from build123d import *

# Parameters (mm, degrees)
F0_R     = 26.4876043929
F1_DEPTH = 14.732
F2_SIZE  = 2.54
F3_R     = 21.3384472315
F4_DEPTH = 3.048
F4_TAPER = 30
F5_R     = 5.08


with BuildPart() as f1:
    # F0 (on Top) → F1 (new body)
    with BuildSketch(Plane.XY):
        Circle(F0_R)
    extrude(amount=F1_DEPTH)

    # F2
    f2_edges = [f1.edges().sort_by_distance(p)[0] for p in [
        (-26.487604, 0, 14.732),
    ]]
    chamfer(f2_edges, length=F2_SIZE)

    # F3 (on face) → F4 (join)
    with BuildSketch(Plane.XY.offset(14.732)):
        Circle(F3_R)
    extrude(amount=F4_DEPTH, taper=F4_TAPER)

    # F5
    f5_edges = [f1.edges().sort_by_distance(p)[0] for p in [
        (-19.578684, 0, 17.78),
    ]]
    fillet(f5_edges, radius=F5_R)


solid = f1.part
Design review of the part built by this model. Coordinates are the model's own, in mm. A direction names the side the tool comes from. Give positions to 0.01 mm unless a question says otherwise; leave off trailing zeros. Loops run counter-clockwise (first coordinate to the right, second up) from the corner with the lowest first, then second, coordinate; pieces in that order, holes last. Notation, with made-up numbers: M -3,-27.5 L 31,-27.5 A20 ccw 31,-18.5 Z; hole C 49.5,-9 d4. An arc over 180 degrees is marked long. One line per question, with ' | ' between items. Start each with the question number.
1. To check wall thickness, follow L1, parallel to Y at x = -0.5, z = 9.75; L2, parallel to Z at x = 6.5, y = -23; L3, parallel to X at y = -15.5, z = 15. State the ranges of each line that lie inside material, in increasing order.
2. Insertion check: P1, Ø6, axis at y = 14.5, z = 15, coming from the +X side; P2, Ø6, axis at x = 5.5, z = 10.5, coming from the -Y side; P3, Ø3, axis at y = 16, z = 11, coming from the -X side. Each pin has a flat end and moves straight along its axis. Give the tip position at first contact, or say it passes through.
3. Add section A-A (x = 0). Write out the cut boundary in (y, z), plus the area to 3 significant figures.
4. Add section C-C (z = 11.5). Write out the cut boundary in (x, y), plus the area to 3 significant figures.
5. For faces 1 (the face through (-3.45, 26.26, 6.01)), 2 (the face through (-20, -9, 14.732)), list the 3-axis set-ups (+Z, -Z, +X, -X, +Y, -Y) from which the entire face can be reached by the end or side of a thin tool; tool diameter is ignored.
Worked out:
1) L1: y = -26.48 to 26.48 | L2: z = 0 to 14.73 | L3: x = -14.44 to 14.44
2) P1: stops at x = 22.84 | P2: stops at y = -26.37 | P3: stops at x = -22.17
3) outline: M -26.49,0 L 26.49,0 L 26.49,12.19 L 23.95,14.73 L 21.34,14.73 L 21.05,15.24 A5.08 ccw 16.65,17.78 L -16.65,17.78 A5.08 ccw -21.05,15.24 L -21.34,14.73 L -23.95,14.73 L -26.49,12.19 Z | area: 896 mm²
4) outline: C 0,0 d52.98 | area: 2,200 mm²
5) face 1: +Z, -Z | face 2: +Z
